from build123d import *

# Parameters (mm, degrees)
F1_DEPTH = 17
F0_W     = 2
F0_H     = 17
F2_DEPTH = 15
F0_W_2   = 30.8
F3_DEPTH = 1
F4_R     = 3
F4_R_2   = 4
F4_R_3   = 2
F5_DEPTH = 2
F6_DEPTH = 25
F8_DEPTH = 16


with BuildPart() as f1:
    # F0 (on Top) → F1 (new body)
    with BuildSketch(Plane.XY):
        with BuildLine():
            Line((-2, 0), (-68.2691728501, 0))
            ThreePointArc((-68.2691728501, 0), (-68.8592199223, -0.1926311546), (-69.221944097, -0.6963110949))
            Line((-69.221944097, -0.6963110949), (-75.5, -20.3926221898))
            ThreePointArc((-75.5, -20.3926221898), (-75.209195197, -22.1800941445), (-73.5944575062, -23))
            Line((-73.5944575062, -23), (-2, -23))
            ThreePointArc((-2, -23), (-0.5857864376, -22.4142135624), (0, -21))
            Line((0, -21), (0, -2))
            ThreePointArc((0, -2), (-0.5857864376, -0.5857864376), (-2, 0))
        make_face()
        with BuildLine():
            ThreePointArc((-67.0294626472, -3.6963110949), (-66.6667384725, -3.1926311546), (-66.0766914003, -3))
            Line((-66.0766914003, -3), (-54.3, -3))
            Line((-54.3, -3), (-52.3, -3))
            Line((-52.3, -3), (-21.5, -3))
            Line((-21.5, -3), (-19.5, -3))
            Line((-19.5, -3), (-4, -3))
            ThreePointArc((-4, -3), (-3.2928932188, -3.2928932188), (-3, -4))
            Line((-3, -4), (-3, -19))
            ThreePointArc((-3, -19), (-3.2928932188, -19.7071067812), (-4, -20))
            Line((-4, -20), (-19.5, -20))
            Line((-19.5, -20), (-21.5, -20))
            Line((-21.5, -20), (-52.3, -20))
            Line((-52.3, -20), (-54.3, -20))
            Line((-54.3, -20), (-70.8578322998, -20))
            ThreePointArc((-70.8578322998, -20), (-71.6652011452, -19.5900470722), (-71.8106035467, -18.6963110949))
            Line((-71.8106035467, -18.6963110949), (-67.0294626472, -3.6963110949))
        make_face(mode=Mode.SUBTRACT)
    extrude(amount=F1_DEPTH)

    # F0 (on Top) → F2 (join)
    with BuildSketch(Plane.XY):
        with Locations((-53.3, -11.5)):
            Rectangle(F0_W, F0_H)
        with Locations((-20.5, -11.5)):
            Rectangle(F0_W, F0_H)
    extrude(amount=F2_DEPTH)

    # F0 (on Top) → F3 (join)
    with BuildSketch(Plane.XY):
        with BuildLine():
            Line((-54.3, -3), (-66.0766914003, -3))
            ThreePointArc((-66.0766914003, -3), (-66.6667384725, -3.1926311546), (-67.0294626472, -3.6963110949))
            Line((-67.0294626472, -3.6963110949), (-71.8106035467, -18.6963110949))
            ThreePointArc((-71.8106035467, -18.6963110949), (-71.6652011452, -19.5900470722), (-70.8578322998, -20))
            Line((-70.8578322998, -20), (-54.3, -20))
            Line((-54.3, -20), (-54.3, -3))
        make_face()
        with Locations((-36.9, -11.5)):
            Rectangle(F0_W_2, F0_H)
        with BuildLine():
            Line((-4, -3), (-19.5, -3))
            Line((-19.5, -3), (-19.5, -20))
            Line((-19.5, -20), (-4, -20))
            ThreePointArc((-4, -20), (-3.2928932188, -19.7071067812), (-3, -19))
            Line((-3, -19), (-3, -4))
            ThreePointArc((-3, -4), (-3.2928932188, -3.2928932188), (-4, -3))
        make_face()
    extrude(amount=F3_DEPTH)

    # F4 (on Top) → F5 (join)
    with BuildSketch(Plane.XY):
        with BuildLine():
            ThreePointArc((24, -12.5858614946), (23.0159698309, -8.2370738953), (19, -6.3))
            Line((19, -6.3), (-36.3860578131, -6.3))
            Line((-36.3860578131, -6.3), (-39.7084973779, -6.3))
            ThreePointArc((-39.7084973779, -6.3), (-38.5513841423, -8.3396204816), (-38.15, -10.65))
            ThreePointArc((-38.15, -10.65), (-47.3103795184, -17.0986158577), (-50.2915026221, -6.3))
            Line((-50.2915026221, -6.3), (-71.0080791799, -6.3))
            Line((-71.0080791799, -6.3), (-76.3035875518, -22.9137386762))
            ThreePointArc((-76.3035875518, -22.9137386762), (-61.5627251362, -42.3229885458), (-56.656298365, -66.1963833943))
            ThreePointArc((-56.656298365, -66.1963833943), (-55.2293521755, -69.7987081167), (-51.6573721204, -71.3))
            Line((-51.6573721204, -71.3), (-10.156298365, -71.3))
            ThreePointArc((-10.156298365, -71.3), (5.9662681641, -65.6697477172), (15.0790057851, -51.2269327109))
            Line((15.0790057851, -51.2269327109), (24, -12.5858614946))
        make_face()
        with Locations((-34.656298365, -61.3)):
            Circle(F4_R, mode=Mode.SUBTRACT)
        with Locations((-14.656298365, -60.3)):
            Circle(F4_R_2, mode=Mode.SUBTRACT)
        with Locations((-34.15, -10.65)):
            Circle(F4_R_3, mode=Mode.SUBTRACT)
        with BuildLine():
            Line((-39.7084973779, -6.3), (-36.3860578131, -6.3))
            ThreePointArc((-36.3860578131, -6.3), (-39.9430740563, -2.4311192976), (-45, -1))
            Line((-45, -1), (-69.3187427266, -1))
            Line((-69.3187427266, -1), (-71.0080791799, -6.3))
            Line((-71.0080791799, -6.3), (-50.2915026221, -6.3))
            ThreePointArc((-50.2915026221, -6.3), (-45, -3.8), (-39.7084973779, -6.3))
        make_face()
    extrude(amount=-F5_DEPTH)

    # F6 (cut): faces of the model
    f6_faces = [f1.faces().sort_by_distance(p)[0] for p in [
        (-45, -10.65, 0),
        (-34.15, -10.65, 0),
    ]]
    extrude(f6_faces, amount=-F6_DEPTH, mode=Mode.SUBTRACT)

    # F7 (on Top) → F8 (join)
    with BuildSketch(Plane.XY):
        with BuildLine():
            Line((-29.5, -68.3), (-10.156298365, -68.3))
            ThreePointArc((-10.156298365, -68.3), (4.0987242542, -63.3219232466), (12.1558955908, -50.5520795479))
            Line((12.1558955908, -50.5520795479), (21.0768898056, -11.9110083316))
            ThreePointArc((21.0768898056, -11.9110083316), (21.1260119747, -11.5846639084), (21.1241694926, -11.2546483401))
            ThreePointArc((21.1241694926, -11.2546483401), (21.0354701794, -11.0733493387), (20.8474362182, -11))
            Line((20.8474362182, -11), (-29.5, -11))
            Line((-29.5, -11), (-29.5, -68.3))
        make_face()
        with BuildLine():
            Line((-10.156298365, -66.3), (-27.5, -66.3))
            Line((-27.5, -66.3), (-27.5, -13))
            Line((-27.5, -13), (18.7728680534, -13))
            Line((18.7728680534, -13), (10.2071554612, -50.1021774392))
            ThreePointArc((10.2071554612, -50.1021774392), (2.8536949809, -61.7567069329), (-10.156298365, -66.3))
        make_face(mode=Mode.SUBTRACT)
        with BuildLine():
            Line((-53.6031346189, -68.3), (-38.1031346189, -68.3))
            Line((-38.1031346189, -68.3), (-38.1031346189, -60.3))
            Line((-38.1031346189, -60.3), (-40.5031346189, -60.3))
            Line((-40.5031346189, -60.3), (-40.5031346189, -65.9))
            Line((-40.5031346189, -65.9), (-51.2102166135, -65.9))
            Line((-51.2102166135, -65.9), (-51.2501856031, -65.886270575))
            ThreePointArc((-51.2501856031, -65.886270575), (-55.5697599064, -42.3552473048), (-68.6864102541, -22.3472173679))
            ThreePointArc((-68.6864102541, -22.3472173679), (-66.0038303781, -15.8365100283), (-64.7912408019, -8.9))
            Line((-64.7912408019, -8.9), (-57.25, -8.9))
            Line((-57.25, -8.9), (-57.25, -10.65))
            ThreePointArc((-57.25, -10.65), (-53.8370668211, -19.1334397505), (-45.5, -22.8897916649))
            ThreePointArc((-45.5, -22.8897916649), (-45.2500520996, -22.8974476503), (-45, -22.9))
            Line((-45, -22.9), (-43.1, -22.9))
            Line((-43.1, -22.9), (-33.2, -22.9))
            Line((-33.2, -22.9), (-33.2, -20.5))
            Line((-33.2, -20.5), (-45, -20.5))
            ThreePointArc((-45, -20.5), (-51.9650017947, -17.6150017947), (-54.85, -10.65))
            Line((-54.85, -10.65), (-54.85, -6.5))
            Line((-54.85, -6.5), (-67.1262612777, -6.5))
            ThreePointArc((-67.1262612777, -6.5), (-68.2643194585, -15.0127044985), (-71.7676746543, -22.8541212502))
            ThreePointArc((-71.7676746543, -22.8541212502), (-58.1079401486, -42.5901979394), (-53.6031346189, -66.1657742205))
            Line((-53.6031346189, -66.1657742205), (-53.6031346189, -68.3))
        make_face()
        with BuildLine():
            Line((-43.1, -28), (-43.1, -22.9))
            Line((-43.1, -22.9), (-45, -22.9))
            ThreePointArc((-45, -22.9), (-45.2500520996, -22.8974476503), (-45.5, -22.8897916649))
            Line((-45.5, -22.8897916649), (-45.5, -28))
            Line((-45.5, -28), (-43.1, -28))
        make_face()
    extrude(amount=-F8_DEPTH)


solid = f1.part
Geometry: final body of the model. Coordinates: model frame, mm. A direction names the side the tool comes from. Coordinates: 2 decimals unless noted, no trailing zeros. Order: outer loops, then holes, each group sorted by start corner. A loop starts at its lowest first (then second) coordinate and runs counter-clockwise, first axis right, second up.
(1) Material intervals for probe 1 along Y at (x, z) = (-40, -14); probe 2 along X at (y, z) = (-10.65, -1.2); probe 3 along X at (y, z) = (-61, -1), sorted ascending.
(2) First-contact query: pin 1 (2.5 mm diameter, centred on y = -67, z = -8, fed in from -X); pin 2 (2 mm diameter, centred on y = -16, z = 6.5, fed in from +X); pin 3 (6 mm diameter, centred on x = 2.5, z = 7.5, fed in from +Y); pin 4 (4 mm diameter, centred on x = -26.5, y = -33, fed in from -Z). Flat tips, straight axial feed; report the tip coordinate or a pass-through.
(3) Section query A-A (x = -13.5). Return the cut outline in (y, z), plus the area to 3 significant figures.
(4) Access query for faces 4 (the face through (-21.5, -12, 8)), 5 (the face through (-40.503, -63, -9)), 6 (the face through (-38, -23, 8)). Directions: +Z, -Z, +X, -X, +Y, -Y. A direction counts if a zero-diameter tool reaches every point of the face in a straight line with its end or side. Return the directions, or none.
(5) Section query B-B (z = -9.5). State how many separate pieces and enclosed holes the cut face has, plus the area to 3 significant figures.
(6) Section query D-D (x = 3.5). Return the cut outline in (y, z).
(7) Section query C-C (y = -42.5). Return the cut outline in (x, z).
(8) Draft query along Y for faces 1 (the face through (-20, -3, 0)), 2 (the face through (-31, -71.3, -1)), 3 (the face through (-35, -3, 9)). Return one class per face: pulls with the +Y half, pulls with the -Y half, needs draft (parallel to the pull), parting line crosses it, or undercut.
Solution:
1. probe 1: y = -68.3 to -60.3, -22.9 to -20.5
1. probe 2: x = -72.39 to -51.85, -38.15 to -36.15, -32.15 to 24.07
1. probe 3: x = -56.79 to -37.64, -31.67 to -18.59, -10.72 to 10.52
2. pin 1: stops at x = -53.6
2. pin 2: stops at x = 0
2. pin 3: stops at y = -0.68
2. pin 4: stops at z = -16
3. outline: (-71.3, -2) - (-68.3, -2) - (-68.3, -16) - (-66.3, -16) - (-66.3, -2) - (-64.13, -2) - (-64.13, 0) - (-71.3, 0) - close; (-56.47, -2) - (-13, -2) - (-13, -16) - (-11, -16) - (-11, -2) - (-6.3, -2) - (-6.3, 0) - (0, 0) - (0, 17) - (-3, 17) - (-3, 1) - (-20, 1) - (-20, 17) - (-23, 17) - (-23, 0) - (-56.47, 0) - close
3. area: 290 mm2
4. face 4: +Z
4. face 5: -Z
4. face 6: +Z, +X, -X, -Y
5. separate pieces: 2
5. enclosed holes: 1
5. area: 700 mm2
6. outline: (-67.41, -2) - (-63.78, -2) - (-63.78, -16) - (-61.22, -16) - (-61.22, -2) - (-13, -2) - (-13, -16) - (-11, -16) - (-11, -2) - (-6.3, -2) - (-6.3, 0) - (-67.41, 0) - close
7. outline: (-61.48, -2) - (-58.15, -2) - (-58.15, -16) - (-55.51, -16) - (-55.51, -2) - (-29.5, -2) - (-29.5, -16) - (-27.5, -16) - (-27.5, -2) - (11.96, -2) - (11.96, -16) - (14.01, -16) - (14.01, -2) - (17.09, -2) - (17.09, 0) - (-61.48, 0) - close
8. face 1: needs draft
8. face 2: pulls with the -Y half
8. face 3: undercut
